Geometry check sheet. Reference: the model listing, model coordinates, mm. A direction names the side the tool comes from. Give positions to 0.01 mm unless a question says otherwise; leave off trailing zeros. Write each loop counter-clockwise with the first axis right and the second up, starting at its lowest first coordinate (ties: lowest second). Pieces come first, ordered by that corner, then holes. Notation, with made-up numbers: M 11.5,-30.75 L 54.5,-30.75 A23 ccw 54.5,-18.75 Z; hole C -18.5,38 d11. An arc over 180 degrees is marked long. Write each question's results on one line, items separated by ' | '.
```python
from build123d import *

# Parameters (mm, degrees)
F1_DEPTH = 30
F2_R     = 5
F3_R     = 5


with BuildPart() as f1:
    # F0 (on Front) → F1 (new body)
    with BuildSketch(Plane.XZ):
        Polygon((-15, 2), (-15, 0), (15, 0), (15, 2), (7.1, 2), (7.1, 15), (5.1, 15), (5.1, 2), (-5.1, 2), (-5.1, 15), (-7.1, 15), (-7.1, 2), align=None)
    extrude(amount=-F1_DEPTH)

    # F2
    f2_edges = [f1.edges().sort_by_distance(p)[0] for p in [
        (-15, 0, 1),
        (15, 0, 1),
        (-15, 30, 1),
        (15, 30, 1),
    ]]
    fillet(f2_edges, radius=F2_R)

    # F3
    f3_edges = [f1.edges().sort_by_distance(p)[0] for p in [
        (-7.1, 15, 2),
        (7.1, 15, 2),
    ]]
    fillet(f3_edges, radius=F3_R)


solid = f1.part
```
Q1. Section check A-A (z = 3). Enter the section's corners in (x, y).
Answer key:
outline: M -9.1,0 L -5.1,0 L -5.1,30 L -9.1,30 Z; M 5.1,0 L 9.1,0 L 9.1,30 L 5.1,30 Z
Q2. Access from +Z, -Z, +X, -X, +Y, -Y to the whole of each face (thin tool, end or side, straight path). Record for faces 1 (the face through (5.1, 15, 9)), 2 (the face through (14, 28, 1)), 3 (the face through (-14, 15, 2)), 4 (the face through (7.1, 15, 11)).
Answer key:
face 1: +Z, +Y, -Y | face 2: +Z, -Z, +X, +Y | face 3: +Z, -X, +Y, -Y | face 4: +Z, +X, +Y, -Y
Q3. Section check D-D (x = -4). Enter the section's corners in (y, z), then the cut area to 3 significant figures.
Answer key:
outline: M 0,0 L 30,0 L 30,2 L 0,2 Z | area: 60.0 mm2
Q4. Release check for a two-part mould opening along X. For faces 5 (the face through (14, 2, 1)), 6 (the face through (0, 15, 2)), 7 (the face through (14, 15, 2)) record: released by +X, released by -X, zero draft, split by the parting line, or undercut.
Answer key:
face 5: released by +X | face 6: undercut | face 7: zero draft
Q5. Material ranges on probe 1 along X at (y, z) = (5.5, 8.5); probe 2 along Z at (x, y) = (1.5, 28); probe 3 along X at (y, z) = (7.5, 3.5), recorded low to high. Write a range as [from, to].
Answer key:
probe 1: x = [-7.1, -5.1], [5.1, 7.1] | probe 2: z = [0, 2] | probe 3: x = [-8.53, -5.1], [5.1, 8.53]
Q6. Section check C-C (z = 9.25). Enter the section's corners in (x, y), then the cut area to 3 significant figures.
Answer key:
outline: M -7.1,0 L -5.1,0 L -5.1,30 L -7.1,30 Z; M 5.1,0 L 7.1,0 L 7.1,30 L 5.1,30 Z | area: 120 mm2
Q7. Section check B-B (y = 23.5). Enter the section's corners in (x, z), then the cut area to 3 significant figures.
Answer key:
outline: M -15,0 L 15,0 L 15,2 L 12.1,2 A5 cw 7.1,7 L 7.1,15 L 5.1,15 L 5.1,2 L -5.1,2 L -5.1,15 L -7.1,15 L -7.1,7 A5 cw -12.1,2 L -15,2 Z | area: 123 mm2
Q8. Depth check by flat-ended pin: P1, Ø2.5, axis at y = 7.5, z = 9, coming from the +X side; P2, Ø3, axis at x = -5, y = 16, coming from the +Z side; P3, Ø6.5, axis at y = 18.5, z = 12, coming from the -X side; P4, Ø0.9, axis at x = 13, y = 15, coming from the +Z side. Enter the tip coordinate at first touch or a pass-through.
Answer key:
P1: stops at x = 7.1 | P2: stops at z = 15 | P3: stops at x = -7.1 | P4: stops at z = 2
